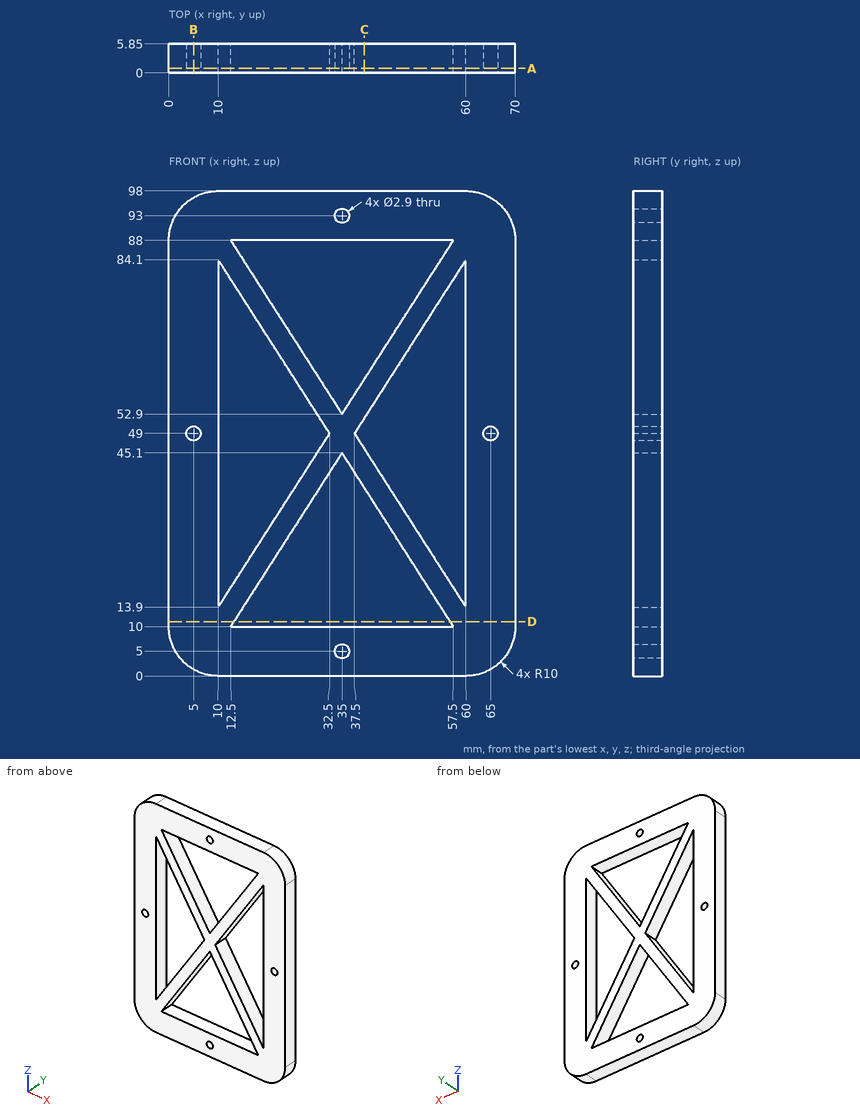
Print and shaded views of the part. All mm, measured from the part's lowest x, y and z. Give positions to 0.01 mm unless a question says otherwise; leave off trailing zeros. Write each loop counter-clockwise with the first axis right and the second up, starting at its lowest first coordinate (ties: lowest second). Pieces come first, ordered by that corner, then holes. Notation, with made-up numbers: (-27, 30) -> (16, 30) arc R26 ccw to (16, 49) -> close; hole circle Ø11 at (-7, 89). An arc over 180 degrees is marked (long way). Write item = value, one per line.
(1) Slice it at D-D, the plane z = 11. Give the cut face in (x, y).
Determined:
outline = (0, 0) -> (13.14, 0) -> (13.14, 5.85) -> (0, 5.85) -> close; (56.86, 0) -> (70, 0) -> (70, 5.85) -> (56.86, 5.85) -> close
(2) Slice it at C-C, the plane x = 39.5. Give the cut face in (y, z).
Determined:
outline = (0, 0) -> (5.85, 0) -> (5.85, 10) -> (0, 10) -> close; (0, 38.08) -> (5.85, 38.08) -> (5.85, 45.88) -> (0, 45.88) -> close; (0, 52.12) -> (5.85, 52.12) -> (5.85, 59.92) -> (0, 59.92) -> close; (0, 88) -> (5.85, 88) -> (5.85, 98) -> (0, 98) -> close
(3) Slice it at B-B, the plane x = 5. Give the cut face in (y, z), then the cut area to 3 significant figures.
Determined:
outline = (0, 1.34) -> (5.85, 1.34) -> (5.85, 47.55) -> (0, 47.55) -> close; (0, 50.45) -> (5.85, 50.45) -> (5.85, 96.66) -> (0, 96.66) -> close
area = 541 mm2
(4) Probe line 1 along X through (y, z) = (1.9, 49); line 2 along Z through (x, y) = (31, 3.95); line 3 along Z through (x, y) = (33, 5.65). List the from-to ranges inside material, lowest first.
Determined:
line_1 = 0 to 3.55, 6.45 to 10, 32.5 to 37.5, 60 to 63.55, 66.45 to 70
line_2 = 0 to 10, 38.86 to 46.66, 51.34 to 59.14, 88 to 98
line_3 = 0 to 10, 41.98 to 56.02, 88 to 98
(5) Slice it at A-A, the plane y = 0.9. Give the number of separate pieces and of enclosed holes in the cut face, then the cut area to 3 significant figures.
Determined:
separate_pieces = 1
enclosed_holes = 8
area = 3,590 mm2
